Read the model definition and answer for the solid it produces. Units are mm, in the model's axes. A direction names the side the tool comes from. Round coordinates to 2 decimals unless told otherwise and drop trailing zeros. Order: outer loops, then holes, each group sorted by start corner. A loop starts at its lowest first (then second) coordinate and runs counter-clockwise, first axis right, second up. Notation, with made-up numbers: M 76.25,10 L 113.25,10 A20 cw 113.25,43 Z; hole C 2,38 d3. An arc over 180 degrees is marked long. Answer as CSV lines item,"result".
```python
from build123d import *

# Parameters (mm, degrees)
SKETCH_1_W          = 20
SKETCH_1_H          = 20
SKETCH_1_W_2        = 18
SKETCH_1_H_2        = 18
EXTRUDE_1_DEPTH     = 740
SKETCH_3_R          = 1.65
CUT_EXTRUDE_1_DEPTH = 32
SKETCH_5_R          = 15.397397092
CUT_EXTRUDE_2_DEPTH = 180
SKETCH_7_R          = 1.65
CUT_EXTRUDE_3_DEPTH = 40


with BuildPart() as part:
    # 草图1 → 凸台-拉伸1 (new body)
    with BuildSketch(Plane(origin=(0, 0, 0), x_dir=(1, 0, 0), z_dir=(0, 1, 0))):
        Rectangle(SKETCH_1_W, SKETCH_1_H)
        Rectangle(SKETCH_1_W_2, SKETCH_1_H_2, mode=Mode.SUBTRACT)
    extrude(amount=EXTRUDE_1_DEPTH)

    # 草图3 → 切除-拉伸1 (cut)
    with BuildSketch(Plane.XY.offset(10)):
        with Locations((0, 720)):
            Circle(SKETCH_3_R)
        with Locations((0, 700)):
            Circle(SKETCH_3_R)
        with Locations((0, 680)):
            Circle(SKETCH_3_R)
        with Locations((0, 660)):
            Circle(SKETCH_3_R)
        with Locations((0, 590)):
            Circle(SKETCH_3_R)
        with Locations((0, 570)):
            Circle(SKETCH_3_R)
        with Locations((0, 550)):
            Circle(SKETCH_3_R)
        with Locations((0, 450)):
            Circle(SKETCH_3_R)
        with Locations((0, 430)):
            Circle(SKETCH_3_R)
        with Locations((0, 410)):
            Circle(SKETCH_3_R)
    extrude(amount=-CUT_EXTRUDE_1_DEPTH, mode=Mode.SUBTRACT)

    # 草图5 → 切除-拉伸2 (cut)
    with BuildSketch(Plane.XZ):
        Circle(SKETCH_5_R)
    extrude(amount=-CUT_EXTRUDE_2_DEPTH, mode=Mode.SUBTRACT)

    # 草图7 → 切除-拉伸3 (cut)
    with BuildSketch(Plane.XY.offset(10)):
        with Locations((0, 190)):
            Circle(SKETCH_7_R)
        with Locations((0, 200)):
            Circle(SKETCH_7_R)
        with Locations((0, 210)):
            Circle(SKETCH_7_R)
        with Locations((0, 310)):
            Circle(SKETCH_7_R)
        with Locations((0, 330)):
            Circle(SKETCH_7_R)
        with Locations((0, 350)):
            Circle(SKETCH_7_R)
    extrude(amount=-CUT_EXTRUDE_3_DEPTH, mode=Mode.SUBTRACT)


solid = part.part
```
Item 1: A tool of negligible diameter and unlimited length cuts with its end or side. For faces 1 (the face through (-10, 456, 0)), 2 (the face through (0, 456, 9)), from which of +Z, -Z, +X, -X, +Y, -Y can it reach the whole face along a straight path? Write none if from no direction.
Ans:
face 1,"+Z, -Z, -X, +Y, -Y"
face 2,"+Y, -Y"
Item 2: A cutting plane is placed at A-A, the plane y = 511. Determine the outline of the cut face in (x, z).
Ans:
outline,"M -10,-10 L 10,-10 L 10,10 L -10,10 Z; hole M -9,-9 L 9,-9 L 9,9 L -9,9 Z"
Item 3: Determine the mould class of faces 3 (the face through (-0.8, 180, -9.6)), 4 (the face through (0, 456, -9)), 5 (the face through (0, 456, -10)), 6 (the face through (-9, 456, 0)) for opening direction Z: +Z half, -Z half, draft (parallel to the pull), parting line (faces both ways), or undercut.
Ans:
face 3,"draft"
face 4,"undercut"
face 5,"-Z half"
face 6,"undercut"
Item 4: A flat-ended cylindrical pin translates along its axis: pin 1 (2 mm diameter, centred on x = 0, y = 310, fed in from -Z). Find the tip coordinate at first contact, or state that the pin passes through.
Ans:
pin 1,"through"
Item 5: A cutting plane is placed at B-B, the plane z = -1.5. Determine the outline of the cut face in (x, y), and give its area (3 significant figures).
Ans:
outline,"M -10,180 L -9,180 L -9,740 L -10,740 Z; M 9,180 L 10,180 L 10,740 L 9,740 Z"
area,"1,120 mm2"
Item 6: Find the intervals of material crossed by probe 1 along Z at (x, y) = (-3.25, 426.5); probe 2 along X at (y, z) = (450, -9.4), in increasing order. Write a range as [from, to].
Ans:
probe 1,"[-10, -9], [9, 10]"
probe 2,"[-10, -1.65], [1.65, 10]"
